```python
from build123d import *

# Parameters (mm, degrees)
F0_W     = 91.686919
F0_H     = 87.288838
F1_DEPTH = 141.779242
F2_SIZE  = 6.35
F3_T     = -2.54


with BuildPart() as f1:
    # F0 (on Front) → F1 (new body)
    with BuildSketch(Plane.XZ):
        with Locations((-45.843459, -43.644419)):
            Rectangle(F0_W, F0_H)
    extrude(amount=F1_DEPTH)

    # F2
    f2_edges = [f1.edges().sort_by_distance(p)[0] for p in [
        (-45.84346, -141.779242, 0),
        (-91.686919, -70.889621, 0),
        (-91.686919, -70.889621, -87.288838),
        (-91.686919, 0, -43.644419),
        (-91.686919, -141.779242, -43.644419),
        (0, -70.889621, 0),
        (-45.84346, 0, 0),
        (-45.84346, -141.779242, -87.288838),
        (0, -141.779242, -43.644419),
        (0, 0, -43.644419),
    ]]
    chamfer(f2_edges, length=F2_SIZE)

    # F3
    f3_openings = [f1.faces().sort_by_distance(p)[0] for p in [
        (-42.739325, -67.829256, -87.288838),
    ]]
    offset(amount=F3_T, openings=f3_openings)


solid = f1.part
```
Verification items for the finished model (mm, model axes). A direction names the side the tool comes from. Give positions to 0.01 mm unless a question says otherwise; leave off trailing zeros. Loops run counter-clockwise (first coordinate to the right, second up) from the corner with the lowest first, then second, coordinate; pieces in that order, holes last. Notation, with made-up numbers: M -30.75,18 L -3.75,18 A23 ccw -3.75,38 Z; hole C -39,67.25 d1. An arc over 180 degrees is marked long. One line per question, with ' | ' between items.
Item 1: Depth check by flat-ended pin: P1, Ø10, axis at x = -12.5, y = -105.5, coming from the -Z side. Enter the tip coordinate at first touch or a pass-through.
Completed:
P1: stops at z = -2.54
Item 2: Thickness scan on line 1 (Y direction, x = -23, z = -67); line 2 (X direction, y = -64, z = -9); line 3 (Z direction, x = -62, y = -129.5). Record the ranges inside material, lowest first. Write a range as [from, to].
Completed:
line 1: y = [-141.78, -139.24], [-2.54, 0] | line 2: x = [-91.69, -89.15], [-2.54, 0] | line 3: z = [-2.54, 0]
Item 3: Section check A-A, the plane x = -48. Record the cut outline in (y, z), plus the area to 3 significant figures.
Completed:
outline: M -141.78,-80.94 L -135.43,-87.29 L -131.84,-87.29 L -139.24,-79.89 L -139.24,-7.4 L -134.38,-2.54 L -7.4,-2.54 L -2.54,-7.4 L -2.54,-87.29 L 0,-87.29 L 0,-6.35 L -6.35,0 L -135.43,0 L -141.78,-6.35 Z | area: 781 mm^2
Item 4: Draft check along Z on faces 1 (the face through (0, -70, -47)), 2 (the face through (-3.93, -137.35, -4.34)), 3 (the face through (-85.394, -67.656, -83.64)). Enter one of: +Z half, -Z half, draft (parallel to the pull), parting line (faces both ways), or undercut.
Completed:
face 1: draft | face 2: +Z half | face 3: undercut
Item 5: Tool access check on faces 4 (the face through (-3.22, -3.13, -47.39)), 5 (the face through (-5.8, -5.5, -5.8)), 6 (the face through (-85.912, -5.487, -5.837)). Record the directions out of +Z, -Z, +X, -X, +Y, -Y that give a thin tool (end or side, any length) a straight path to the whole face; none if there is none.
Completed:
face 4: +Z, -Z, +X, +Y | face 5: -Z | face 6: none
Item 6: Section check B-B, the plane z = -12. Record the cut outline in (x, y).
Completed:
outline: M -91.69,-135.43 L -85.34,-141.78 L -6.35,-141.78 L 0,-135.43 L 0,-6.35 L -6.35,0 L -85.34,0 L -91.69,-6.35 Z; hole M -89.15,-134.38 L -84.28,-139.24 L -7.4,-139.24 L -2.54,-134.38 L -2.54,-7.4 L -7.4,-2.54 L -84.28,-2.54 L -89.15,-7.4 Z
Item 7: Section check C-C, the plane y = -112. Record the cut outline in (x, z), plus the area to 3 significant figures.
Completed:
outline: M -91.69,-80.94 L -85.34,-87.29 L -81.74,-87.29 L -89.15,-79.89 L -89.15,-7.4 L -84.28,-2.54 L -7.4,-2.54 L -2.54,-7.4 L -2.54,-87.29 L 0,-87.29 L 0,-6.35 L -6.35,0 L -85.34,0 L -91.69,-6.35 Z | area: 654 mm^2
